Verification items for the finished model (mm, model axes). Face numbers are marked on the shaded views. A direction names the side the tool comes from. Round coordinates to 2 decimals unless told otherwise and drop trailing zeros. Order: outer loops, then holes, each group sorted by start corner. A loop starts at its lowest first (then second) coordinate and runs counter-clockwise, first axis right, second up. Notation, with made-up numbers: M 54.5,-19.75 L 67.5,-19.75 A25 ccw 67.5,4.25 Z; hole C 36,-35 d10. An arc over 180 degrees is marked long. One line per item, written item: value. Start each with the question number.
Autodesk Inventor part; units mm, degrees
ref_plane "Work Plane1" through (0, 0, 0) normal (0, -1, 0) x (1, 0, 0)
ref_plane "Work Plane2" through (0, 0, -22.86) normal (0, 0, 1) x (1, 0, 0)
ref_plane "YZ Plane" through (0, 0, 0) normal (1, 0, 0) x (0, 1, 0)
sketch "Sketch1" plane through (0, 0, 0) normal (0, 1, 0) x (-1, 0, 0)
  circle A0 centre (0, 0) radius 43.18
  dimension "d0" = 86.36
extrude "Extrusion1" add sketch "Sketch1" against normal blind 63.5
sketch "Sketch2" plane through (0, 0, 0) normal (0, 0, 1) x (1, 0, 0)
  line L0 (-43.18, 0) -> (43.18, 0)
  arc A0 (-43.18, 0) -> (43.18, 0) centre (0, 24.003) ccw
  line L1 (-43.18, -63.5) -> (43.18, -63.5)
  point P0 (0, 0)
  dimension "d4" = 38.1
extrude "Extrusion2" cut sketch "Sketch2" along normal mid plane 101.6
ref_plane "Work Plane1" through (0, 0, 0) normal (0, -1, 0) x (1, 0, 0)
sketch "Sketch3" plane through (0, 0, 0) normal (0, -1, 0) x (1, 0, 0)
  circle A0 centre (0, 0) radius 38.1
  dimension "d8" = 76.2
extrude "Extrusion3" cut sketch "Sketch3" along normal blind 57.15
sketch "Sketch4" plane through (0, 0, 0) normal (1, 0, 0) x (0, 1, 0)
  circle A0 centre (-25.4, 0) radius 12.7
  point P0 (0, 0)
  dimension "d11" = 25.4
  dimension "d12" = 25.4
  dimension "d13" = 0
extrude "Extrusion4" add sketch "Sketch4" along normal mid plane 78.74
sketch "Sketch5" plane through (0, 0, 0) normal (1, 0, 0) x (0, 1, 0)
  circle A0 centre (-25.4, 0) radius 13.97
  arc A1 (-25.4, 17.145) -> (-25.4, -17.145) centre (-25.4, 0) ccw
  line L0 (-63.5, 43.18) -> (-63.5, -43.18)
  circle A2 centre (93.98, 0) radius 20.32
  arc A3 (90.484, -25.1583) -> (93.98, 25.4) centre (93.98, 0) ccw
  line L1 (93.98, 25.4) -> (-25.4, 17.145)
  line L2 (90.484, -25.1583) -> (-25.4, -17.145)
  point P0 (0, 0)
  point P1 (-25.4, 12.7)
  dimension "d16" = 27.94
  dimension "d17" = 34.29
  dimension "d18" = 38.1
  dimension "d19" = 43.18
  dimension "d20" = 40.64
  dimension "d21" = 0
  dimension "d22" = 119.38
  dimension "d23" = 50.8
extrude "Extrusion5" add sketch "Sketch5" along normal mid plane 31.75
sketch "Sketch6" plane through (0, 0, 0) normal (1, 0, 0) x (0, 1, 0)
  circle A0 centre (93.98, 0) radius 20.32 construction
  line L0 (93.98, 0) -> (93.98, -43.5701)
  line L1 (93.98, 0) -> (93.98, 40.9183)
  line L2 (93.98, 40.9183) -> (142.8926, 40.9183)
  line L3 (142.8926, 40.9183) -> (133.2711, -47.8298)
  line L4 (133.2711, -47.8298) -> (93.98, -43.5701)
  point P0 (0, 0)
extrude "Extrusion6" cut sketch "Sketch6" along normal mid plane 2540
ref_plane "Work Plane2" through (0, 0, -22.86) normal (0, 0, 1) x (1, 0, 0)
sketch "Sketch7" plane through (0, 0, -22.86) normal (0, 0, 1) x (1, 0, 0)
  line L0 (15.875, 90.484) -> (15.875, 93.98)
  line L1 (-15.875, -25.4) -> (-15.875, 93.98) construction
  line L2 (15.875, 93.98) -> (-15.875, 93.98)
  line L3 (-15.875, 93.98) -> (-15.875, 88.9)
  line L4 (-15.875, 88.9) -> (15.875, 88.9)
  line L5 (15.875, 88.9) -> (15.875, 93.98)
  point P0 (0, 0)
  dimension "d29" = 5.08
extrude "Extrusion7" add sketch "Sketch7" against normal blind 6.35
mirror "Mirror1" about plane through (0, 0, 0) normal (0, 0, 1) of "Extrusion7"
sketch "Sketch8" plane through (15.875, 0, 0) normal (1, 0, 0) x (0, 0, -1)
  circle A0 centre (0, -25.4) radius 13.97
  line L0 (-20.32, 93.98) -> (-29.21, 93.98)
  arc A1 (-20.32, 93.98) -> (20.32, 93.98) centre (0, 93.98) ccw
  line L1 (20.32, 93.98) -> (29.21, 93.98)
  line L2 (29.21, 88.9) -> (29.21, 93.98)
  line L3 (25.0487, 88.9) -> (29.21, 88.9)
  line L4 (25.0487, 88.9) -> (17.145, -25.4)
  arc A2 (-17.145, -25.4) -> (17.145, -25.4) centre (0, -25.4) ccw
  line L5 (-17.145, -25.4) -> (-25.0487, 88.9)
  line L6 (-25.0487, 88.9) -> (-29.21, 88.9)
  line L7 (-29.21, 88.9) -> (-29.21, 93.98)
  point P0 (0, 0)
extrude "Extrusion8" cut sketch "Sketch8" against normal blind 38.1
properties part number "PistonsHead"
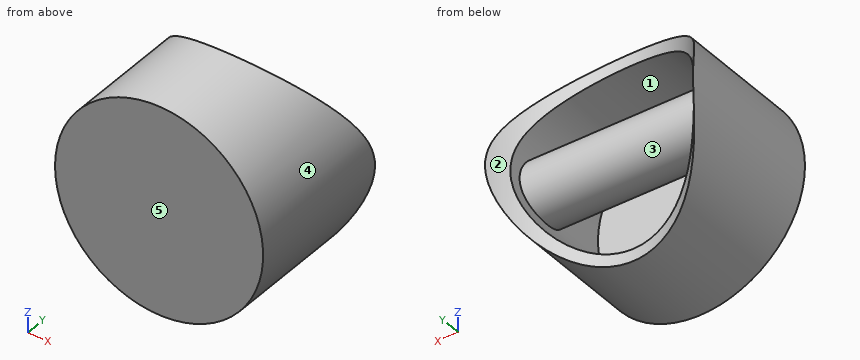
1. Tool access check on the marked faces 1 and 2. Record the directions out of +Z, -Z, +X, -X, +Y, -Y that give a thin tool (end or side, any length) a straight path to the whole face; none if there is none.
2. Section check C-C (y = -41). Record the cut outline in (x, z), and give its area (3 significant figures).
3. Scan lines: line 1 along Z through (x, y) = (0, -44); line 2 along Z through (x, y) = (0, -31); line 3 along Y through (x, z) = (-14.5, -31.5). Record each from-to range of solid material in increasing order.
4. Section check A-A (x = 0). Record the cut outline in (y, z).
5. Section check B-B (z = 0). Record the cut outline in (x, y).
6. Depth check by flat-ended pin: pin 1 (1 mm diameter, centred on x = 23, y = -39, fed in from +Z); pin 2 (2 mm diameter, centred on x = 10, y = -40.5, fed in from -Z); pin 3 (5 mm diameter, centred on x = 20.5, y = -39.5, fed in from +Z). Enter the tip coordinate at first touch or a pass-through.
7. Section check D-D (z = 16). Record the cut outline in (x, y), and give its area (3 significant figures).
8. Draft check along Z on the marked faces 3, 4 and 5. Enter one of: released by +Z, released by -Z, zero draft, split by the parting line, or undercut.
Geometry check:
1. face 1: none
1. face 2: +Y
2. outline: C 0,0 d86.36; hole C 0,0 d76.2
2. area: 1,300 mm²
3. line 1: z = -43.18 to -38.1, 38.1 to 43.18
3. line 2: z = -43.18 to -38.1, -11.4 to 11.4, 38.1 to 43.18
3. line 3: y = -63.5 to -57.15
4. outline: M -63.5,-43.18 L -25.4,-43.18 L -25.4,-38.1 L -57.15,-38.1 L -57.15,38.1 L -25.4,38.1 L -25.4,43.18 L -63.5,43.18 Z; C -25.4,0 d25.4
5. outline: M -43.18,-63.5 L 43.18,-63.5 L 43.18,0 A49.4 cw 38.1,-7.45 L 38.1,-12.7 L -38.1,-12.7 L -38.1,-7.45 A49.4 cw -43.18,0 Z; hole M -38.1,-57.15 L 38.1,-57.15 L 38.1,-38.1 L -38.1,-38.1 Z
6. pin 1: stops at z = 36.85
6. pin 2: stops at z = -42.23
6. pin 3: stops at z = 39.25
7. outline: M -40.11,-63.5 L 40.11,-63.5 L 40.11,-4.84 A49.4 cw 34.58,-11.28 L 34.58,-57.15 L -34.58,-57.15 L -34.58,-11.28 A49.4 cw -40.11,-4.84 Z
7. area: 1,050 mm²
8. face 3: undercut
8. face 4: split by the parting line
8. face 5: zero draft
